Autodesk Inventor part; units mm, degrees
ref_plane "YZ Plane" through (0, 0, 0) normal (1, 0, 0) x (0, 1, 0)
ref_plane "XZ Plane" through (0, 0, 0) normal (0, 1, 0) x (-1, 0, 0)
ref_plane "XY Plane" through (0, 0, 0) normal (0, 0, 1) x (1, 0, 0)
sketch "Esquisse1" plane through (0, 0, 0) normal (0, 1, 0) x (-1, 0, 0)
  line L0 (0, 0) -> (32, 0) construction
  line L1 (32, 0) -> (16, 27.7128) construction
  line L2 (16, 27.7128) -> (0, 0) construction
  line L3 (-10.3913, 17.9982) -> (9.0252, -15.6322) construction
  line L4 (8, -13.8564) -> (32, 0) construction
  line L5 (8, -13.8564) -> (14.9282, -9.8564) construction
  line L6 (8, -13.8564) -> (-10, 17.3205) construction
  line L7 (-10, 17.3205) -> (1.6913, 24.0705) construction
  line L8 (1.6913, 24.0705) -> (4.9413, 18.4413) construction
  line L9 (4.9413, 18.4413) -> (8.9413, 11.5131) construction
  line L10 (8.9413, 11.5131) -> (12.9413, 4.5849) construction
  line L11 (12.9413, 4.5849) -> (16.9413, -2.3433) construction
  circle A0 centre (8.9413, 11.5131) radius 1
  circle A1 centre (12.9413, 4.5849) radius 1
  circle A2 centre (16.9413, -2.3433) radius 1
  circle A3 centre (14.9282, -9.8564) radius 1
  circle A4 centre (4.9413, 18.4413) radius 1
  circle A5 centre (-14.4413, -1.9869) radius 1 construction
  circle A6 centre (-10.4413, -8.9151) radius 1
  circle A7 centre (-6.4413, -15.8433) radius 1
  circle A8 centre (1.0718, -17.8564) radius 1
  circle A9 centre (-18.4413, 4.9413) radius 1 construction
  circle A10 centre (-10, 17.3205) radius 11.6 construction
  line L12 (32, 0) -> (36, -6.9282) construction
  line L13 (36.0415, 0) -> (34.0207, -3.5) construction
  line L14 (34.0207, -3.5) -> (29.9793, -3.5) construction
  line L15 (29.9793, -3.5) -> (27.9585, 0) construction
  line L16 (27.9585, 0) -> (29.9793, 3.5) construction
  line L17 (29.9793, 3.5) -> (34.0207, 3.5) construction
  line L18 (34.0207, 3.5) -> (36.0415, 0) construction
  line L19 (34.0207, 3.5) -> (34.0207, -3.5) construction
  circle A11 centre (16, 27.7128) radius 2
  circle A12 centre (32, 0) radius 2
  line L20 (32, 0) -> (38.9282, 4) construction
  line L21 (-6.4413, -15.8433) -> (-13.3695, -19.8433) construction
  line L22 (42.9282, -2.9282) -> (-6.6195, -31.5346)
  line L23 (-6.6195, -31.5346) -> (-30.6195, 10.0346)
  line L24 (-30.6195, 10.0346) -> (18.9282, 38.641)
  line L25 (18.9282, 38.641) -> (42.9282, -2.9282)
  line L26 (8, -13.8564) -> (12, -20.7846) construction
  line L27 (16, 27.7128) -> (12, 34.641) construction
  circle A13 centre (0, 0) radius 2
  dimension "d0" = 32
  dimension "d1" = 32
  dimension "d2" = 60
  dimension "d4" = 8
  dimension "d6" = 36
  dimension "d7" = 13.5
  dimension "d8" = 6.5
  dimension "d9" = 8
  dimension "d10" = 8
  dimension "d11" = 8
  dimension "d13" = 2
  dimension "d14" = 11.6
  dimension "d15" = 8
  dimension "d16" = 7
  dimension "d17" = 4
  dimension "d19" = 8
  dimension "d20" = 8
  dimension "d26" = 8
  dimension "d27" = 8
extrude "Extrusion4" add sketch "Esquisse1" along normal blind 12
sketch "Esquisse7" plane through (0, 12, 0) normal (0, 1, 0) x (1, 0, 0)
  circle A0 centre (10.4413, 8.9151) radius 1
  circle A1 centre (-4.9413, -18.4413) radius 1
  line L0 (-18.9282, -38.641) -> (30.6195, -10.0346)
  line L1 (30.6195, -10.0346) -> (6.6195, 31.5346)
  line L2 (-4.9413, -18.4413) -> (-1.6913, -24.0705) construction
  line L3 (-1.6913, -24.0705) -> (10, -17.3205) construction
  circle A2 centre (10, -17.3205) radius 12 construction
  line L4 (10.4413, 8.9151) -> (12.4413, 5.451) construction
  line L5 (-0.3923, -23.3205) -> (1.6077, -26.7846)
  line L6 (17.7305, 12.2898) -> (0.5077, -9.9791)
  arc A3 (0.5077, -9.9791) -> (-0.3923, -23.3205) centre (10, -17.3205) ccw
  dimension "d54" = 6.5
  dimension "d55" = 13.5
  dimension "d56" = 24
  dimension "d57" = 4
extrude "Extrusion5" cut sketch "Esquisse7" against normal through all contours L5 A3 L6 L1 L0
fillet "Congé8" radius 10 1 edges at (1.6077, 6, 26.7846)
fillet "Congé9" radius 10 1 edges at (17.7305, 6, -12.2898)
fillet "Congé10" radius 10 1 edges at (6.6195, 6, -31.5346)
fillet "Congé11" radius 10 1 edges at (-42.9282, 6, -2.9282)
fillet "Congé12" radius 10 1 edges at (-18.9282, 6, 38.641)
sketch "Esquisse8" plane through (0, 12, 0) normal (0, 1, 0) x (1, 0, 0)
  circle A0 centre (0, 0) radius 2
  circle A1 centre (-32, 0) radius 2
  circle A2 centre (-16, -27.7128) radius 2
  circle A3 centre (6.4413, 15.8433) radius 1
  circle A4 centre (10.4413, 8.9151) radius 1
  line L0 (-2.0407, 26.5346) -> (-34.2679, 7.9282)
  line L1 (-28.5, 2.0207) -> (-28.5, -2.0207)
  line L2 (-28.5, -2.0207) -> (-32, -4.0415)
  line L3 (-32, -4.0415) -> (-35.5, -2.0207)
  line L4 (-35.5, -2.0207) -> (-35.5, 2.0207)
  line L5 (-35.5, 2.0207) -> (-32, 4.0415)
  line L6 (-32, 4.0415) -> (-28.5, 2.0207)
  line L7 (-19.5, -25.6921) -> (-16, -23.6714)
  line L8 (-16, -23.6714) -> (-12.5, -25.6921)
  line L9 (-12.5, -25.6921) -> (-12.5, -29.7335)
  line L10 (-12.5, -29.7335) -> (-16, -31.7543)
  line L11 (-16, -31.7543) -> (-19.5, -29.7335)
  line L12 (-19.5, -29.7335) -> (-19.5, -25.6921)
  line L13 (-32, 4.0415) -> (-28.5, -2.0207) construction
  line L14 (0, 4.0415) -> (3.5, 2.0207)
  line L15 (3.5, 2.0207) -> (3.5, -2.0207)
  line L16 (3.5, -2.0207) -> (0, -4.0415)
  line L17 (0, -4.0415) -> (-3.5, -2.0207)
  line L18 (-3.5, -2.0207) -> (-3.5, 2.0207)
  line L19 (-3.5, 2.0207) -> (0, 4.0415)
  dimension "d66" = 7
extrude "Extrusion6" cut sketch "Esquisse8" against normal blind 3 contours L1 L2 L3 L4 L5 L6 | L7 L8 L9 L10 L11 L12 | L14 L15 L16 L17 L18 L19
properties part number "joint3+ax12imprint_v2"
Here's how the part is built. I have some questions about the finished solid (model axes, mm). A direction names the side the tool comes from. Round coordinates to 2 decimals unless told otherwise and drop trailing zeros. Loops run counter-clockwise (first coordinate to the right, second up) from the corner with the lowest first, then second, coordinate; pieces in that order, holes last.
1. For faces 4 (the face through (-14.27, 10.52, 24.67)), 5 (the face through (15.7, 5.92, -12.51)), which set-ups out of +Z, -Z, +X, -X, +Y, -Y let a thin tool reach every point of the face, with its end or its side?
Answers:
face 4: +Y
face 5: +X, +Y, -Y
2. Will these pins go through, and if not, where does the flat tip stop? pin 1 (3.5 mm diameter, centred on y = 11, z = 1, fed in from -X); pin 2 (2.5 mm diameter, centred on y = 10.5, z = 27.5, fed in from +X); pin 3 (2 mm diameter, centred on x = -31.5, z = 2, fed in from +Y); pin 4 (4 mm diameter, centred on x = 4.5, y = 5.5, fed in from +Z).
Answers:
pin 1: stops at x = -39.27
pin 2: stops at x = -1.98
pin 3: stops at y = 9
pin 4: stops at z = 7.4
3. Suppose I cut it at B-B, the plane y = 4.5. Give the number of separate pieces and of enclosed holes in the cut face, and give its area (3 significant figures).
Answers:
separate pieces: 1
enclosed holes: 11
area: 1,970 mm2
4. Suppose I cut it at A-A, the plane z = 1. Please give me the cut outline in (x, y).
Answers:
outline: (-39.26, 0) - (-33.73, 0) - (-33.73, 9) - (-35.5, 9) - (-35.5, 12) - (-39.26, 12) - close; (-30.27, 0) - (-1.73, 0) - (-1.73, 9) - (-3.5, 9) - (-3.5, 12) - (-28.5, 12) - (-28.5, 9) - (-30.27, 9) - close; (1.73, 0) - (7.45, 0) - (7.45, 12) - (3.5, 12) - (3.5, 9) - (1.73, 9) - close
5. Suppose I cut it at C-C, the plane x = -23. Please give me the cut outline in (y, z).
Answers:
outline: (0, -14.43) - (12, -14.43) - (12, 31.32) - (0, 31.32) - close
6. If I drill on probe 1 along X at (y, z) = (8.5, -1); probe 2 along X at (y, z) = (10.5, -2); probe 3 along Z at (x, y) = (-13, 11.75), over which ranges is the centre line in solid material (lowest first)?
Answers:
probe 1: x = -39.12 to -33.73, -30.27 to -1.73, 1.73 to 9
probe 2: x = -38.89 to -35.5, -28.5 to -17.88, -16 to -3.5, 3.5 to 9.77
probe 3: z = -20.21 to 3.59, 5.58 to 25.4, 30.02 to 34.72
7. Thinking about a two-plate mould opening in Z: for faces 1 (the face through (-18.38, 5.92, -17.1)), 2 (the face through (-8.272, 5.916, 32.488)), 3 (the face through (-1.726, 10.521, 3.045)), which applies, released by +Z, released by -Z, zero draft, split by the parting line, or undercut?
Answers:
face 1: released by -Z
face 2: released by +Z
face 3: undercut
